from build123d import *

# Parameters (mm, degrees)
ESQUISSE1_R                  = 18
BOSS_EXTRU_2_DEPTH           = 2.75
ESQUISSE2_R                  = 15.915
BOSS_EXTRU_3_DEPTH           = 9
ESQUISSE3_R                  = 18
BOSS_EXTRU_4_DEPTH           = 2.75
ESQUISSE4_R                  = 11.5
BOSS_EXTRU_5_DEPTH           = 8
ESQUISSE5_R                  = 3
ENL_V_MAT_EXTRU_1_DEPTH      = 23.5
ESQUISSE6_R                  = 4
ENL_V_MAT_EXTRU_2_DEPTH      = 10
ESQUISSE7_R                  = 1.35
ENL_V_MAT_EXTRU_3_DEPTH      = 23.5
R_P_TITION_CIRCULAIRE1_COUNT = 8


with BuildPart() as part:
    # Esquisse1 → Boss.-Extru.2 (new body)
    with BuildSketch(Plane.XY):
        Circle(ESQUISSE1_R)
    extrude(amount=BOSS_EXTRU_2_DEPTH)

    # Esquisse2 → Boss.-Extru.3 (add)
    with BuildSketch(Plane.XY.offset(2.75)):
        Circle(ESQUISSE2_R)
    extrude(amount=BOSS_EXTRU_3_DEPTH)

    # Esquisse3 → Boss.-Extru.4 (add)
    with BuildSketch(Plane.XY.offset(11.75)):
        Circle(ESQUISSE3_R)
    extrude(amount=BOSS_EXTRU_4_DEPTH)

    # Esquisse4 → Boss.-Extru.5 (add)
    with BuildSketch(Plane(origin=(0, 0, 0), x_dir=(-1, 0, 0), z_dir=(0, 0, -1))):
        with Locations(Location((0, 0, 0), (0, 0, 180))):  # turned: the seam where the file's is
            Circle(ESQUISSE4_R)
    extrude(amount=BOSS_EXTRU_5_DEPTH)

    # Esquisse5 → Enlèv. mat.-Extru.1 (cut, through all)
    with BuildSketch(Plane(origin=(0, 0, -8), x_dir=(-1, 0, 0), z_dir=(0, 0, -1))):
        Circle(ESQUISSE5_R)
    extrude(amount=-ENL_V_MAT_EXTRU_1_DEPTH, mode=Mode.SUBTRACT)

    # Esquisse6 → Enlèv. mat.-Extru.2 (cut)
    with BuildSketch(Plane(origin=(0, 0, -8), x_dir=(-1, 0, 0), z_dir=(0, 0, -1))):
        Circle(ESQUISSE6_R)
    extrude(amount=-ENL_V_MAT_EXTRU_2_DEPTH, mode=Mode.SUBTRACT)

    # Esquisse7 → Enlèv. mat.-Extru.3 (cut, through all)
    with BuildSketch(Plane(origin=(0, 0, -8), x_dir=(-1, 0, 0), z_dir=(0, 0, -1))):
        with Locations((3.354474935, 7.26274727)):
            Circle(ESQUISSE7_R)
    enl_v_mat_extru_3 = extrude(amount=-ENL_V_MAT_EXTRU_3_DEPTH, mode=Mode.SUBTRACT)

    # Répétition circulaire1: Enlèv. mat.-Extru.3 ×8 about axis
    r_p_tition_circulaire1_axis = Axis((0, 0, 0), (0, 0, 1))
    for i in range(1, R_P_TITION_CIRCULAIRE1_COUNT):
        add(enl_v_mat_extru_3.rotate(r_p_tition_circulaire1_axis, i * 360 / R_P_TITION_CIRCULAIRE1_COUNT), mode=Mode.SUBTRACT)


solid = part.part
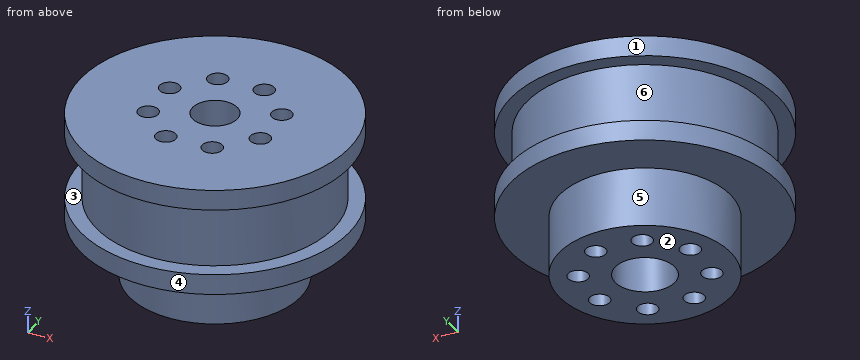
Work out the finished part from the listing and answer in its coordinate system (mm). Face numbers are marked on the shaded views. A direction names the side the tool comes from. Round coordinates to 2 decimals unless told otherwise and drop trailing zeros. Write each loop counter-clockwise with the first axis right and the second up, starting at its lowest first coordinate (ties: lowest second). Pieces come first, ordered by that corner, then holes. Notation, with made-up numbers: (84, 6.25) -> (138, 6.25) arc R20 ccw to (138, 37.25) -> close; hole circle Ø7 at (58, 79). An arc over 180 degrees is marked (long way). Answer as CSV lines item,"result". Start each with the question number.
(1) The part is cut by section A-A, the plane x = 0. Give the vertices of the cut face in (y, z) (3 decimals).
(2) A tool of negligible diameter and unlimited length cuts with its end or side. For the marked faces 4, 5 and 6, from which of +Z, -Z, +X, -X, +Y, -Y can it reach the whole face along a straight path? Write none if from no direction.
(3) Find the intervals of material crossed by probe 1 along Y at (x, z) = (0, -1); probe 2 along X at (y, z) = (3.5, 13.5); probe 3 along X at (y, z) = (-7, 8.75), in increasing order.
(4) The part is cut by section D-D, the plane x = 12.5. Give the vertices of the cut face in (y, z).
(5) Each of these flat-tipped pins is pushed along its axis until it touches: pin 1 (4 mm diameter, centred on x = 3, y = -2, fed in from -Z); pin 2 (3 mm diameter, centred on x = 0, z = -2, fed in from +Y); pin 3 (1 mm diameter, centred on x = -7.5, z = -2, fed in from +Y); pin 4 (6 mm diameter, centred on y = -7, z = 7, fed in from +X). Where does it stop, or does it pass through?
(6) The part is cut by section C-C, the plane z = -4. Give the number of separate pieces and of enclosed holes in the cut face, then the cut area to 3 significant figures.
(7) The mould has two halves that part along Z. Classify the marked faces 1, 2 and 3: +Z half, -Z half, draft (parallel to the pull), parting line (faces both ways), or undercut.
Output values:
1,outline,"(-18, 0) -> (-11.5, 0) -> (-11.5, -8) -> (-4, -8) -> (-4, 2) -> (-3, 2) -> (-3, 14.5) -> (-18, 14.5) -> (-18, 11.75) -> (-15.915, 11.75) -> (-15.915, 2.75) -> (-18, 2.75) -> close; (3, 2) -> (4, 2) -> (4, -8) -> (11.5, -8) -> (11.5, 0) -> (18, 0) -> (18, 2.75) -> (15.915, 2.75) -> (15.915, 11.75) -> (18, 11.75) -> (18, 14.5) -> (3, 14.5) -> close"
2,face 4,"+Z, -Z"
2,face 5,"-Z"
2,face 6,"none"
3,probe 1,"y = -11.5 to -4, 4 to 11.5"
3,probe 2,"x = -17.66 to -8.64, -6.38 to 5.92, 8.6 to 17.66"
3,probe 3,"x = -14.29 to -4.01, -1.51 to 2.03, 4.68 to 14.29"
4,outline,"(-12.95, 0) -> (12.95, 0) -> (12.95, 2.75) -> (9.85, 2.75) -> (9.85, 11.75) -> (12.95, 11.75) -> (12.95, 14.5) -> (-12.95, 14.5) -> (-12.95, 11.75) -> (-9.85, 11.75) -> (-9.85, 2.75) -> (-12.95, 2.75) -> close"
5,pin 1,"stops at z = -8"
5,pin 2,"stops at y = 11.5"
5,pin 3,"stops at y = 9.12"
5,pin 4,"stops at x = 15.4"
6,separate pieces,"1"
6,enclosed holes,"9"
6,area,"319 mm²"
7,face 1,"draft"
7,face 2,"-Z half"
7,face 3,"undercut"
